from build123d import *

# Parameters (mm, degrees)
BOSS_EXTRUDE1_DEPTH    = 30
FILLET1_R              = 0.254
LPATTERN1_COUNT        = 10
LPATTERN1_PITCH        = 6.8834
FILLET1_OF_LPATTERN1_R = 0.254


with BuildPart() as part:
    # Sketch1 → Boss-Extrude1 (new, symmetric)
    with BuildSketch(Plane.XY):
        with BuildLine():
            Line((0, 0), (1.22, 0))
            ThreePointArc((1.22, 0), (3.76, 4.945446374), (6.3, 0))
            Line((6.3, 0), (7.52, 0))
            Line((7.52, 0), (7.52, 5.580446374))
            Line((7.52, 5.580446374), (0, 5.580446374))
            Line((0, 5.580446374), (0, 0))
        make_face()
    boss_extrude1 = extrude(amount=BOSS_EXTRUDE1_DEPTH, both=True)

    # Fillet1
    fillet1_edges = [part.edges().sort_by_distance(p)[0] for p in [
        (6.3, 0, 0),
        (1.22, 0, 0),
    ]]
    fillet(fillet1_edges, radius=FILLET1_R)

    # LPattern1: Boss-Extrude1 ×10
    with Locations(*[(-i * LPATTERN1_PITCH, 0, 0) for i in range(1, LPATTERN1_COUNT)]):
        add(boss_extrude1)

    # Fillet1 of LPattern1
    fillet1_of_lpattern1_edges = [part.edges().sort_by_distance(p)[0] for p in [
        (-0.5834, 0, 0),
        (-5.6634, 0, 0),
        (-7.4668, 0, 0),
        (-12.5468, 0, 0),
        (-14.3502, 0, 0),
        (-19.4302, 0, 0),
        (-21.2336, 0, 0),
        (-26.3136, 0, 0),
        (-28.117, 0, 0),
        (-33.197, 0, 0),
        (-35.0004, 0, 0),
        (-40.0804, 0, 0),
        (-41.8838, 0, 0),
        (-46.9638, 0, 0),
        (-48.7672, 0, 0),
        (-53.8472, 0, 0),
        (-55.6506, 0, 0),
        (-60.7306, 0, 0),
    ]]
    fillet(fillet1_of_lpattern1_edges, radius=FILLET1_OF_LPATTERN1_R)


solid = part.part
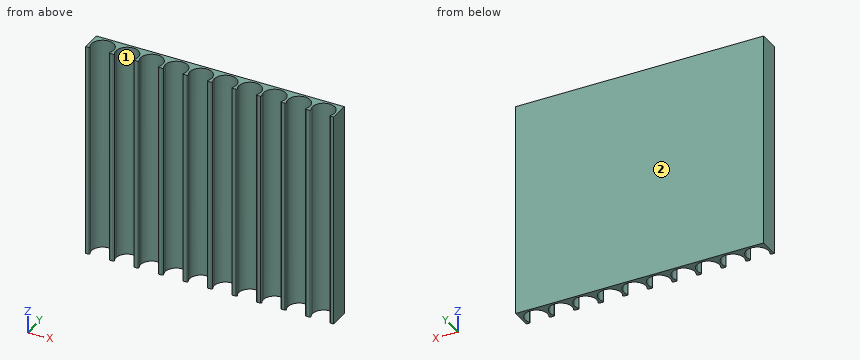
Here's how the part is built. I have some questions about the finished solid (model axes, mm). Face numbers are marked on the shaded views. Coordinates: 2 decimals unless noted, no trailing zeros. Order: outer loops, then holes, each group sorted by start corner. A loop starts at its lowest first (then second) coordinate and runs counter-clockwise, first axis right, second up. Notation, with made-up numbers: (12, 19.25) - (37, 19.25) arc R21 ccw to (37, 55.25) - close; hole circle Ø10 at (33.25, -13). An arc over 180 degrees is marked (long way). Use CSV: the item, a comma, the result in double quotes. Start each with the question number.
1. If we mould it in two halves opening along Y, with no side actions, what happens to the marked faces 1 and 2? For each: +Y half, -Y half, draft (parallel to the pull), parting line (faces both ways), or undercut.
2. Please list where these lines run through material, in increasing order: line 1 (Y direction, x = 3.76, z = -10.5); line 2 (Y direction, x = -8, z = 12). Write a range as from..to.
3. Suppose I cut it at B-B on y = 3.1. Give the number of separate pieces and of enclosed holes in the cut face, then the cut area to 3 significant figures.
4. Suppose I cut it at A-A on x = 3.76. List the corners of the cut face in (y, z) for me, then the cut area to 3 significant figures.
5. Suppose I cut it at C-C on x = -43.5. List the corners of the cut face in (y, z) for me, then the cut area to 3 significant figures.
6. I'm going to push a flat-ended pin straight in: pin 1 (2 mm diameter, centred on x = -23, z = 17, fed in from -Y). Where does the tip first touch, or does it pass through?
Output:
1,face 1,"undercut"
1,face 2,"+Y half"
2,line 1,"y = 4.95..5.58"
2,line 2,"y = 4.22..5.58"
3,separate pieces,"11"
3,enclosed holes,"0"
3,area,"747 mm2"
4,outline,"(4.95, -30) - (5.58, -30) - (5.58, 30) - (4.95, 30) - close"
4,area,"38.1 mm2"
5,outline,"(4.81, -30) - (5.58, -30) - (5.58, 30) - (4.81, 30) - close"
5,area,"46.5 mm2"
6,pin 1,"stops at y = 4.39"
